CAD build for the part. Positions are in the model's coordinates, mm. Face numbers are marked on the shaded views. A direction names the side the tool comes from. Round coordinates to 2 decimals unless told otherwise and drop trailing zeros. Write each loop counter-clockwise with the first axis right and the second up, starting at its lowest first coordinate (ties: lowest second). Pieces come first, ordered by that corner, then holes. Notation, with made-up numbers: M -21,-40 L -3,-40 A34 cw -3,-5 Z; hole C 36.25,-16 d5. An arc over 180 degrees is marked long. Write each question's results on one line, items separated by ' | '. Start each with the question number.
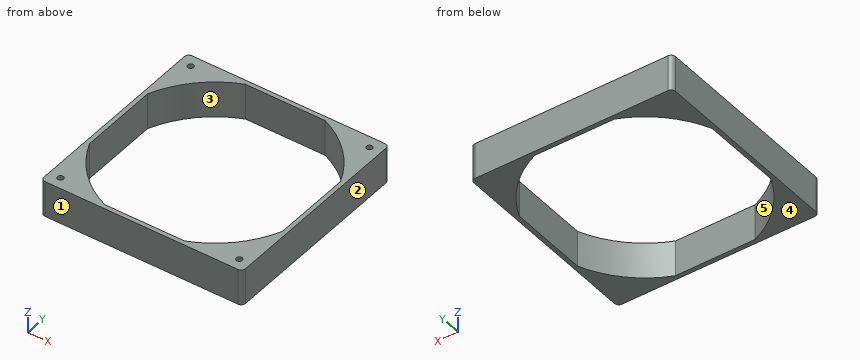
Autodesk Inventor part; units mm, degrees
ref_plane "YZ Plane" through (0, 0, 0) normal (1, 0, 0) x (0, 1, 0)
ref_plane "XZ Plane" through (0, 0, 0) normal (0, 1, 0) x (-1, 0, 0)
ref_plane "XY Plane" through (0, 0, 0) normal (0, 0, 1) x (1, 0, 0)
sketch "Sketch1" plane through (0, 0, 0) normal (0, 0, 1) x (1, 0, 0)
  line L0 (-67, -70) -> (67, -70)
  line L1 (70, -67) -> (70, 67)
  line L2 (67, 70) -> (-67, 70)
  line L3 (-70, 67) -> (-70, -67)
  line L4 (-70, -70) -> (70, 70) construction
  line L5 (70, -70) -> (-70, 70) construction
  arc A0 (-67, 70) -> (-70, 67) centre (-67, 67) ccw
  arc A1 (-70, -67) -> (-67, -70) centre (-67, -67) ccw
  arc A2 (67, -70) -> (70, -67) centre (67, -67) ccw
  arc A3 (70, 67) -> (67, 70) centre (67, 67) ccw
  line L6 (-62.1, -62.1) -> (62.1, -62.1) construction
  line L7 (62.1, -62.1) -> (62.1, 62.1) construction
  line L8 (62.1, 62.1) -> (-62.1, 62.1) construction
  line L9 (-62.1, 62.1) -> (-62.1, -62.1) construction
  line L10 (-62.1, -62.1) -> (62.1, 62.1) construction
  line L11 (62.1, -62.1) -> (-62.1, 62.1) construction
  line L12 (-27.6993, 67) -> (27.6993, 67)
  line L13 (67, 27.6993) -> (67, -27.6993)
  line L14 (27.6993, -67) -> (-27.6993, -67)
  line L15 (-67, -27.6993) -> (-67, 27.6993)
  arc A4 (67, 27.6993) -> (27.6993, 67) centre (0, 0) ccw
  arc A5 (27.6993, -67) -> (67, -27.6993) centre (0, 0) ccw
  arc A6 (-27.6993, 67) -> (-67, 27.6993) centre (0, 0) ccw
  arc A7 (-67, -27.6993) -> (-27.6993, -67) centre (0, 0) ccw
  point P0 (0, 0)
  point P1 (51.2652, -51.2652)
  point P2 (-51.2652, 51.2652)
  dimension "d0" = 140
  dimension "d1" = 140
  dimension "d2" = 3
  dimension "d3" = 124.2
  dimension "d4" = 124.2
  dimension "d6" = 145
  dimension "d7" = 134
extrude "Extrusion1" add sketch "Sketch1" along normal mid plane 25
hole "Hole1" at (-62.1, 62.1, 0) at (62.1, 62.1, 0) at (62.1, -62.1, 0) at (-62.1, -62.1, 0) direction (0, 0, 1) diameter 4.134 end through all
properties part number "nf-a14"
1) Pull direction Y, two halves, no side cores. Call the marked faces 1, 2 and 3: pulls with the +Y half, pulls with the -Y half, needs draft (parallel to the pull), parting line crosses it, or undercut.
2) Drop a flat-ended pin along its axis: pin 1 Ø1.2 at (x, y) = (61.5, 62) entering from +Z. Give the stop position or say it passes through.
3) Wall check: line 1 along Y through (x, z) = (-62.1, 4.5); line 2 along X through (y, z) = (-22, 2.5). Give the ranges that are in metal, low to high. Write a range as from..to.
4) Saw through at D-D, the plane z = -5. Write the cut outline in (x, y).
5) Saw through at B-B, the plane z = 9. Write the cut outline in (x, y).
6) Saw through at A-A, the plane y = 20. Write the cut outline in (x, z).
7) 3-axis set-ups, long thin cutter, end or side, ignore diameter. For the marked faces 4 and 5: which of +Z, -Z, +X, -X, +Y, -Y reach the whole face in a straight line?
Filled sheet:
1) face 1: pulls with the -Y half | face 2: needs draft | face 3: undercut
2) pin 1: stops at z = 0
3) line 1: y = -70..-64.17, -60.03..-37.41, 37.41..60.03, 64.17..70 | line 2: x = -70..-67, 67..70
4) outline: M -70,-67 A3 ccw -67,-70 L 67,-70 A3 ccw 70,-67 L 70,67 A3 ccw 67,70 L -67,70 A3 ccw -70,67 Z; hole M -67,-27.7 A72.5 ccw -27.7,-67 L 27.7,-67 A72.5 ccw 67,-27.7 L 67,27.7 A72.5 ccw 27.7,67 L -27.7,67 A72.5 ccw -67,27.7 Z
5) outline: M -70,-67 A3 ccw -67,-70 L 67,-70 A3 ccw 70,-67 L 70,67 A3 ccw 67,70 L -67,70 A3 ccw -70,67 Z; hole M -67,-27.7 A72.5 ccw -27.7,-67 L 27.7,-67 A72.5 ccw 67,-27.7 L 67,27.7 A72.5 ccw 27.7,67 L -27.7,67 A72.5 ccw -67,27.7 Z; hole C -62.1,-62.1 d4.13; hole C -62.1,62.1 d4.13; hole C 62.1,-62.1 d4.13; hole C 62.1,62.1 d4.13
6) outline: M -70,-12.5 L -67,-12.5 L -67,12.5 L -70,12.5 Z; M 67,-12.5 L 70,-12.5 L 70,12.5 L 67,12.5 Z
7) face 4: -Z, +X, -X, +Y, -Y | face 5: +Z, -Z
